```python
from build123d import *

# Parameters (mm, degrees)
SKETCH1_W           = 146.05
SKETCH1_H           = 50.8
BOSS_EXTRUDE1_DEPTH = 58.42
SHELL1_T            = -5.08
SKETCH2_W           = 50.8
SKETCH2_H           = 5.08
CUT_EXTRUDE2_DEPTH  = 5.08
SKETCH4_W           = 38.1
SKETCH4_H           = 50.8
CUT_EXTRUDE3_DEPTH  = 6.35


with BuildPart() as part:
    # Sketch1 → Boss-Extrude1 (new body)
    with BuildSketch(Plane(origin=(0, 0, 0), x_dir=(1, 0, 0), z_dir=(0, 1, 0))):
        with Locations((73.025, 25.4)):
            Rectangle(SKETCH1_W, SKETCH1_H)
    extrude(amount=BOSS_EXTRUDE1_DEPTH)

    # Shell1
    shell1_openings = [part.faces().sort_by_distance(p)[0] for p in [
        (73.025, 58.42, -25.4),
    ]]
    offset(amount=SHELL1_T, openings=shell1_openings, kind=Kind.INTERSECTION)

    # Sketch2 → Cut-Extrude2 (cut)
    with BuildSketch(Plane.XY):
        with Locations((73.025, 2.54)):
            Rectangle(SKETCH2_W, SKETCH2_H)
        with BuildLine():
            ThreePointArc((98.425, 5.08), (73.025, 30.48), (47.625, 5.08))
            Line((47.625, 5.08), (98.425, 5.08))
        make_face()
    extrude(amount=-CUT_EXTRUDE2_DEPTH, mode=Mode.SUBTRACT)

    # Sketch4 → Cut-Extrude3 (cut)
    with BuildSketch(Plane(origin=(0, 58.42, 0), x_dir=(1, 0, 0), z_dir=(0, 1, 0))):
        with Locations((73.025, 25.4)):
            Rectangle(SKETCH4_W, SKETCH4_H)
    extrude(amount=-CUT_EXTRUDE3_DEPTH, mode=Mode.SUBTRACT)


solid = part.part
```
Here's how the part is built. I have some questions about the finished solid (model axes, mm). A direction names the side the tool comes from. Coordinates: 2 decimals unless noted, no trailing zeros. Order: outer loops, then holes, each group sorted by start corner. A loop starts at its lowest first (then second) coordinate and runs counter-clockwise, first axis right, second up.
1) Imagine slicing it at D-D on x = 89. List the corners of the cut face in (y, z) for me, and give its area (3 significant figures).
2) We'd pull the mould along Z, two halves only. Please class faces 5 (the face through (4.9, 58.42, -25.5)), 6 (the face through (72, 35, 0)), 7 (the face through (72, 31, -5.08)): +Z half, -Z half, draft (parallel to the pull), parting line (faces both ways), or undercut.
3) Imagine slicing it at B-B on x = 111. List the corners of the cut face in (y, z) for me, and give its area (3 significant figures).
4) Imagine slicing it at A-A on y = 43. List the corners of the cut face in (x, z) for me.
5) Which directions (+Z, -Z, +X, -X, +Y, -Y) give clear straight access to the entire face, cutting with the end or side of a thin tool? Please do faces 1 (the face through (98.425, 3, -3)), 2 (the face through (53.975, 55, -3)), 3 (the face through (143, 58.42, -27)), 4 (the face through (72, 31, -45.72)).
6) Imagine slicing it at C-C on z = -43. List the corners of the cut face in (x, y) for me.
7) I need wall thicknesses on line 1 (Z direction, x = 74, y = 41); line 2 (X direction, y = 51.5, z = -31); line 3 (Y direction, x = 34, z = -29). Which ranges of each line are inside material? Lowest first, please.
8) Will these pins go through, and if not, where does the flat tip stop? pin 1 (1.5 mm diameter, centred on x = 70.5, z = -47.5, fed in from +Y); pin 2 (12 mm diameter, centred on x = 85, z = -20, fed in from +Y); pin 3 (2.5 mm diameter, centred on x = 79.5, y = 1.5, fed in from +Z).
Response values:
1. outline: (0, -50.8) - (52.07, -50.8) - (52.07, -45.72) - (5.08, -45.72) - (5.08, -5.08) - (0, -5.08) - close; (24.83, -5.08) - (52.07, -5.08) - (52.07, 0) - (24.83, 0) - close
1. area: 609 mm2
2. face 5: draft
2. face 6: +Z half
2. face 7: undercut
3. outline: (0, -50.8) - (58.42, -50.8) - (58.42, -45.72) - (5.08, -45.72) - (5.08, -5.08) - (58.42, -5.08) - (58.42, 0) - (0, 0) - close
3. area: 800 mm2
4. outline: (0, -50.8) - (146.05, -50.8) - (146.05, 0) - (0, 0) - close; hole (5.08, -45.72) - (140.97, -45.72) - (140.97, -5.08) - (5.08, -5.08) - close
5. face 1: +Z, -Y
5. face 2: +Z, -Z, +Y
5. face 3: +Z, -Z, +X, -X, +Y
5. face 4: +Y
6. outline: (0, 0) - (146.05, 0) - (146.05, 58.42) - (140.97, 58.42) - (140.97, 5.08) - (5.08, 5.08) - (5.08, 58.42) - (0, 58.42) - close
7. line 1: z = -50.8 to -45.72, -5.08 to 0
7. line 2: x = 0 to 5.08, 140.97 to 146.05
7. line 3: y = 0 to 5.08
8. pin 1: stops at y = 52.07
8. pin 2: stops at y = 5.08
8. pin 3: stops at z = -5.08
